```python
from build123d import *

# Parameters (mm, degrees)
SKETCH1_R           = 12.5
BOSS_EXTRUDE1_DEPTH = 57
SKETCH2_R           = 7
CUT_EXTRUDE1_DEPTH  = 60
SKETCH3_W           = 18
SKETCH3_H           = 32
CUT_EXTRUDE2_DEPTH  = 30
BOSS_EXTRUDE2_START = 2.9
SKETCH4_W           = 50
SKETCH4_H           = 152.4
SKETCH4_R           = 2.25
BOSS_EXTRUDE2_DEPTH = 5.1
BOSS_EXTRUDE3_START = 2
BOSS_EXTRUDE3_DEPTH = 10
SKETCH6_R           = 7
BOSS_EXTRUDE4_DEPTH = 6
SKETCH7_R           = 1.5
CUT_EXTRUDE3_DEPTH  = 14


with BuildPart() as part:
    # Sketch1 → Boss-Extrude1 (new, symmetric)
    with BuildSketch(Plane.XY):
        with Locations(Location((0, 7, 0), (0, 0, 180))):
            Circle(SKETCH1_R)
    extrude(amount=BOSS_EXTRUDE1_DEPTH, both=True)

    # Sketch2 → Cut-Extrude1 (cut, symmetric)
    with BuildSketch(Plane.XY):
        with Locations((0, 7)):
            Circle(SKETCH2_R)
    extrude(amount=CUT_EXTRUDE1_DEPTH, both=True, mode=Mode.SUBTRACT)

    # Sketch3 → Cut-Extrude2 (cut, symmetric)
    with BuildSketch(Plane(origin=(0, 0, 0), x_dir=(1, 0, 0), z_dir=(0, 1, 0))):
        Rectangle(SKETCH3_W, SKETCH3_H)
    extrude(amount=CUT_EXTRUDE2_DEPTH, both=True, mode=Mode.SUBTRACT)

    # Sketch4 → Boss-Extrude2 (add)
    with BuildSketch(Plane(origin=(0, 0, 0), x_dir=(1, 0, 0), z_dir=(0, 1, 0)).offset(BOSS_EXTRUDE2_START)):
        with Locations((35, 0)):
            Rectangle(SKETCH4_W, SKETCH4_H)
        with Locations(Location((37.1, 69.05, 0), (0, 0, 270))):
            Circle(SKETCH4_R, mode=Mode.SUBTRACT)
        with Locations(Location((37.1, 61.9935, 0), (0, 0, 270))):
            Circle(SKETCH4_R, mode=Mode.SUBTRACT)
        with Locations(Location((37.1, 54.937, 0), (0, 0, 270))):
            Circle(SKETCH4_R, mode=Mode.SUBTRACT)
        with Locations(Location((37.1, 47.8805, 0), (0, 0, 270))):
            Circle(SKETCH4_R, mode=Mode.SUBTRACT)
        with Locations(Location((37.1, 40.824, 0), (0, 0, 270))):
            Circle(SKETCH4_R, mode=Mode.SUBTRACT)
        with Locations(Location((37.1, 33.7675, 0), (0, 0, 270))):
            Circle(SKETCH4_R, mode=Mode.SUBTRACT)
        with Locations(Location((37.1, 26.711, 0), (0, 0, 270))):
            Circle(SKETCH4_R, mode=Mode.SUBTRACT)
        with Locations(Location((37.1, 19.6545, 0), (0, 0, 270))):
            Circle(SKETCH4_R, mode=Mode.SUBTRACT)
        with Locations(Location((37.1, 12.598, 0), (0, 0, 270))):
            Circle(SKETCH4_R, mode=Mode.SUBTRACT)
        with Locations(Location((37.1, 5.5415, 0), (0, 0, 270))):
            Circle(SKETCH4_R, mode=Mode.SUBTRACT)
        with Locations(Location((37.1, -1.515, 0), (0, 0, 270))):
            Circle(SKETCH4_R, mode=Mode.SUBTRACT)
        with Locations(Location((37.1, -8.5715, 0), (0, 0, 270))):
            Circle(SKETCH4_R, mode=Mode.SUBTRACT)
        with Locations(Location((37.1, -15.628, 0), (0, 0, 270))):
            Circle(SKETCH4_R, mode=Mode.SUBTRACT)
        with Locations(Location((37.1, -22.6845, 0), (0, 0, 270))):
            Circle(SKETCH4_R, mode=Mode.SUBTRACT)
        with Locations(Location((37.1, -29.741, 0), (0, 0, 270))):
            Circle(SKETCH4_R, mode=Mode.SUBTRACT)
        with Locations(Location((37.1, -36.7975, 0), (0, 0, 270))):
            Circle(SKETCH4_R, mode=Mode.SUBTRACT)
        with Locations(Location((37.1, -43.854, 0), (0, 0, 270))):
            Circle(SKETCH4_R, mode=Mode.SUBTRACT)
        with Locations(Location((37.1, -50.9105, 0), (0, 0, 270))):
            Circle(SKETCH4_R, mode=Mode.SUBTRACT)
        with Locations(Location((37.1, -57.967, 0), (0, 0, 270))):
            Circle(SKETCH4_R, mode=Mode.SUBTRACT)
        with Locations(Location((37.1, -65.0235, 0), (0, 0, 270))):
            Circle(SKETCH4_R, mode=Mode.SUBTRACT)
    extrude(amount=BOSS_EXTRUDE2_DEPTH)

    # Sketch5 → Boss-Extrude3 (add)
    with BuildSketch(Plane(origin=(0, 0, 0), x_dir=(1, 0, 0), z_dir=(0, 1, 0)).offset(BOSS_EXTRUDE3_START)):
        Polygon((-9, 15.68), (-9, 18.68), (-80, 5.77), (-80, 2.77), align=None)
        Polygon((-9, -15.68), (-9, -18.68), (-80, -5.77), (-80, -2.77), align=None)
    extrude(amount=BOSS_EXTRUDE3_DEPTH)

    # Sketch6 → Boss-Extrude4 (add, symmetric)
    with BuildSketch(Plane.XY):
        with Locations(Location((-80, 7, 0), (0, 0, 45.584691403))):
            Circle(SKETCH6_R)
    extrude(amount=BOSS_EXTRUDE4_DEPTH, both=True)

    # Sketch7 → Cut-Extrude3 (cut, symmetric)
    with BuildSketch(Plane(origin=(0, 0, 0), x_dir=(1, 0, 0), z_dir=(0, 1, 0))):
        with Locations(Location((-75.5, 0, 0), (0, 0, 270))):
            Circle(SKETCH7_R)
    extrude(amount=CUT_EXTRUDE3_DEPTH, both=True, mode=Mode.SUBTRACT)


solid = part.part
```
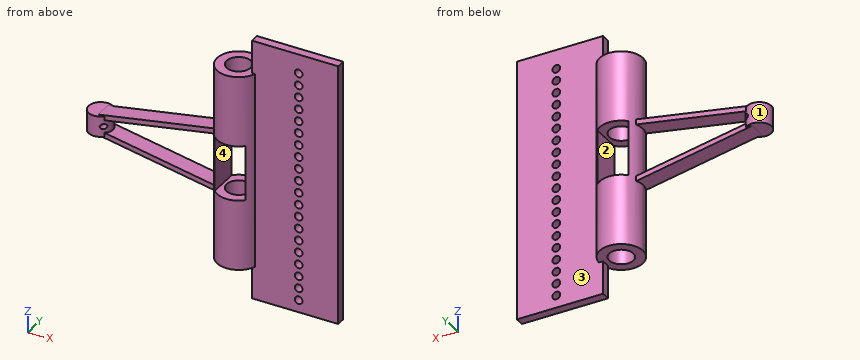
Design review of the part built by this model. Coordinates are the model's own, in mm. Face numbers are marked on the shaded views. A direction names the side the tool comes from. Round coordinates to 2 decimals unless told otherwise and drop trailing zeros. Order: outer loops, then holes, each group sorted by start corner. A loop starts at its lowest first (then second) coordinate and runs counter-clockwise, first axis right, second up. Notation, with made-up numbers: M 42,-8 L 93,-8 A17 cw 93,9 Z; hole C 42,76.25 d9. An arc over 180 degrees is marked long. Put each result on its own line as item: value.
Q1. Insertion check: pin 1 Ø16 at (x, z) = (-34, 11) entering from +Y; pin 2 Ø2.5 at (y, z) = (5, 66.5) entering from -X; pin 3 Ø12 at (x, y) = (-6.5, 4.5) entering from +Z. Each pin has a flat end and moves straight along its axis. Give the tip position at first contact, or say it passes through.
Reported:
pin 1: y = 12
pin 2: x = 10
pin 3: z = 57
Q2. Draft analysis for pull direction Z (two halves, no side actions). For the marked faces 3 and 4, state which applies: released by +Z, released by -Z, zero draft, split by the parting line, or undercut.
Reported:
face 3: zero draft
face 4: undercut
Q3. Consider section D-D (x = -39). State the section outline as (y, z) points, and give its area (3 significant figures).
Reported:
outline: M 2,-13.23 L 12,-13.23 L 12,-10.23 L 2,-10.23 Z; M 2,10.23 L 12,10.23 L 12,13.23 L 2,13.23 Z
area: 60.0 mm²
Q4. Consider section B-B (z = -69.05). State the section outline as (x, y) points.
Reported:
outline: M 10,2.9 L 34.85,2.9 L 34.85,8 L 10,8 Z; M 39.35,2.9 L 60,2.9 L 60,8 L 39.35,8 Z
Q5. Consider section C-C (x = 0). State the section outline as (y, z) points, and give its area (3 significant figures).
Reported:
outline: M -5.5,-57 L 0,-57 L 0,-16 L -5.5,-16 Z; M -5.5,16 L 0,16 L 0,57 L -5.5,57 Z; M 14,-57 L 19.5,-57 L 19.5,-16 L 14,-16 Z; M 14,16 L 19.5,16 L 19.5,57 L 14,57 Z
area: 902 mm²
Q6. To check wall thickness, follow line 1 (Y direction, x = 0, z = 53.5); line 2 (Y direction, x = 14, z = 55.5); line 3 (X direction, y = 4.25, z = 49). State the ranges of each line that lie inside material, in increasing order.
Reported:
line 1: -5.5 to 0, 14 to 19.5
line 2: 2.9 to 8
line 3: -12.19 to -6.44, 6.44 to 35.91, 38.29 to 60
Q7. Consider section A-A (y = 9.75). State the section outline as (x, z) points.
Reported:
outline: M -86.44,-6 L -78.74,-6 L -12.19,-18.1 L -12.19,-57 L -6.44,-57 L -6.44,-16 L -9,-16 L -9,16 L -6.44,16 L -6.44,57 L -12.19,57 L -12.19,18.1 L -78.74,6 L -86.44,6 Z; M 6.44,-57 L 12.19,-57 L 12.19,57 L 6.44,57 L 6.44,16 L 9,16 L 9,-16 L 6.44,-16 Z; hole C -75.5,0 d3; hole M -73.56,-3.94 L -12.19,-15.1 L -12.19,15.1 L -73.56,3.94 Z
Q8. Machinability: for the marked faces 1 and 2, which of the approach directions +Z, -Z, +X, -X, +Y, -Y give a long, thin tool a straight path to every point of the face, cutting with its end or side? Answer none if there is none.
Reported:
face 1: none
face 2: +Y, -Y
